from build123d import *

# Parameters (mm, degrees)
SKETCH1_W           = 40
SKETCH1_H           = 20
BOSS_EXTRUDE1_DEPTH = 37.5
SKETCH2_W           = 20
SKETCH2_H           = 2
BOSS_EXTRUDE2_DEPTH = 7.5
SKETCH3_W           = 20
SKETCH3_H           = 2
BOSS_EXTRUDE3_DEPTH = 7.5
SKETCH4_R           = 1.75
BOSS_EXTRUDE4_DEPTH = 6


with BuildPart() as part:
    # Sketch1 → Boss-Extrude1 (new body)
    with BuildSketch(Plane(origin=(0, 0, 0), x_dir=(1, 0, 0), z_dir=(0, 1, 0))):
        with Locations((20, -10)):
            Rectangle(SKETCH1_W, SKETCH1_H)
    extrude(amount=BOSS_EXTRUDE1_DEPTH)

    # Sketch2 → Boss-Extrude2 (add)
    with BuildSketch(Plane(origin=(40, 0, 0), x_dir=(0, 0, -1), z_dir=(1, 0, 0))):
        with Locations((-10, 31.5)):
            Rectangle(SKETCH2_W, SKETCH2_H)
    extrude(amount=BOSS_EXTRUDE2_DEPTH)

    # Sketch3 → Boss-Extrude3 (add)
    with BuildSketch(Plane.ZY):
        with Locations((10, 31.5)):
            Rectangle(SKETCH3_W, SKETCH3_H)
    extrude(amount=BOSS_EXTRUDE3_DEPTH)

    # Sketch4 → Boss-Extrude4 (add)
    with BuildSketch(Plane(origin=(0, 37.5, 0), x_dir=(1, 0, 0), z_dir=(0, 1, 0))):
        with Locations(Location((32, -10, 0), (0, 0, 270))):
            Circle(SKETCH4_R)
    extrude(amount=BOSS_EXTRUDE4_DEPTH)


solid = part.part
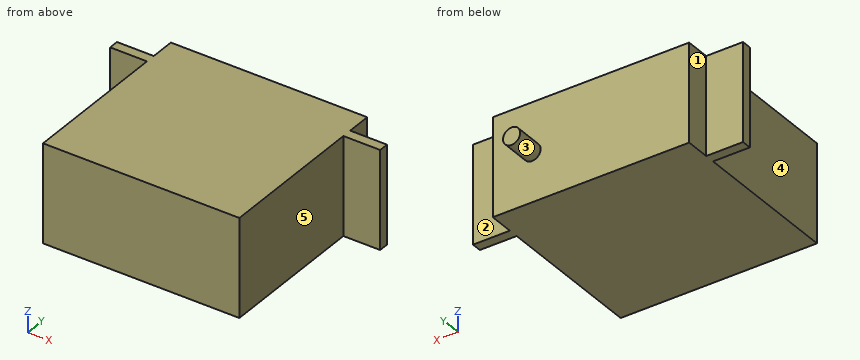
The model under review builds one solid part; all positions refer to its coordinate system, in mm. Face numbers are marked on the shaded views. A direction names the side the tool comes from. Round coordinates to 2 decimals unless told otherwise and drop trailing zeros. Write each loop counter-clockwise with the first axis right and the second up, starting at its lowest first coordinate (ties: lowest second). Pieces come first, ordered by that corner, then holes. Notation, with made-up numbers: (85, 34) - (111, 34) arc R17 cw to (111, 58) - close; hole circle Ø9 at (77, 47). An arc over 180 degrees is marked (long way). One line per item, written item: value. Start each with the question number.
1. Consider section C-C on y = 9. Write out the cut boundary in (x, z), and give its area (3 significant figures).
2. Consider section A-A on x = 32. Write out the cut boundary in (y, z).
3. Machinability: for the marked faces 1, 2, 3, 4 and 5, which of the approach directions +Z, -Z, +X, -X, +Y, -Y give a long, thin tool a straight path to every point of the face, cutting with its end or side? Answer none if there is none.
4. Clearance check with flat-ended pins moving along their axes: P1, Ø1, axis at x = 31.5, z = 16.5, coming from the -Y side; P2, Ø2, axis at x = -3.5, z = 10, coming from the +Y side; P3, Ø3, axis at x = 1, z = 3, coming from the +Y side; P4, Ø4, axis at x = 42.5, z = 7, coming from the -Y side. State where each tip first meets the part, or that it passes through.
5. Consider section D-D on z = 2. Write out the cut boundary in (x, y), and give its area (3 significant figures).
6. Consider section B-B on z = 10. Write out the cut boundary in (x, y), and give its area (3 significant figures).
7. To check wall thickness, follow L1, parallel to Y at x = 21.5, z = 15.5; L2, parallel to X at y = 12, z = 6.25; L3, parallel to Y at x = 43, z = 14. State the ranges of each line that lie inside material, in increasing order. Write a range as from..to.
Checks:
1. outline: (0, 0) - (40, 0) - (40, 20) - (0, 20) - close
1. area: 800 mm^2
2. outline: (0, 0) - (37.5, 0) - (37.5, 8.25) - (43.5, 8.25) - (43.5, 11.75) - (37.5, 11.75) - (37.5, 20) - (0, 20) - close
3. face 1: +Z, -Z, -X, +Y
3. face 2: +Z, -Z, +X, +Y
3. face 3: +Y
3. face 4: +Z, -Z, -X, -Y
3. face 5: +Z, -Z, +X, -Y
4. P1: stops at y = 0
4. P2: stops at y = 32.5
4. P3: stops at y = 37.5
4. P4: stops at y = 30.5
5. outline: (-7.5, 30.5) - (0, 30.5) - (0, 0) - (40, 0) - (40, 30.5) - (47.5, 30.5) - (47.5, 32.5) - (40, 32.5) - (40, 37.5) - (0, 37.5) - (0, 32.5) - (-7.5, 32.5) - close
5. area: 1,530 mm^2
6. outline: (-7.5, 30.5) - (0, 30.5) - (0, 0) - (40, 0) - (40, 30.5) - (47.5, 30.5) - (47.5, 32.5) - (40, 32.5) - (40, 37.5) - (33.75, 37.5) - (33.75, 43.5) - (30.25, 43.5) - (30.25, 37.5) - (0, 37.5) - (0, 32.5) - (-7.5, 32.5) - close
6. area: 1,550 mm^2
7. L1: y = 0..37.5
7. L2: x = 0..40
7. L3: y = 30.5..32.5
